Study the drawing (mm; zero at the part's minimum x, y, z) and answer. A direction names the side the tool comes from. Coordinates: 2 decimals unless noted, no trailing zeros. Write each loop counter-clockwise with the first axis right and the second up, starting at its lowest first coordinate (ties: lowest second). Pieces come first, ordered by that corner, then holes. Notation, with made-up numbers: (84.25, 75.25) -> (88.25, 75.25) arc R15 cw to (88.25, 81.25) -> close; hole circle Ø4 at (77, -17). An arc over 180 degrees is marked (long way). Write each question's results on one line, items separated by ' | '. Start each with the question number.
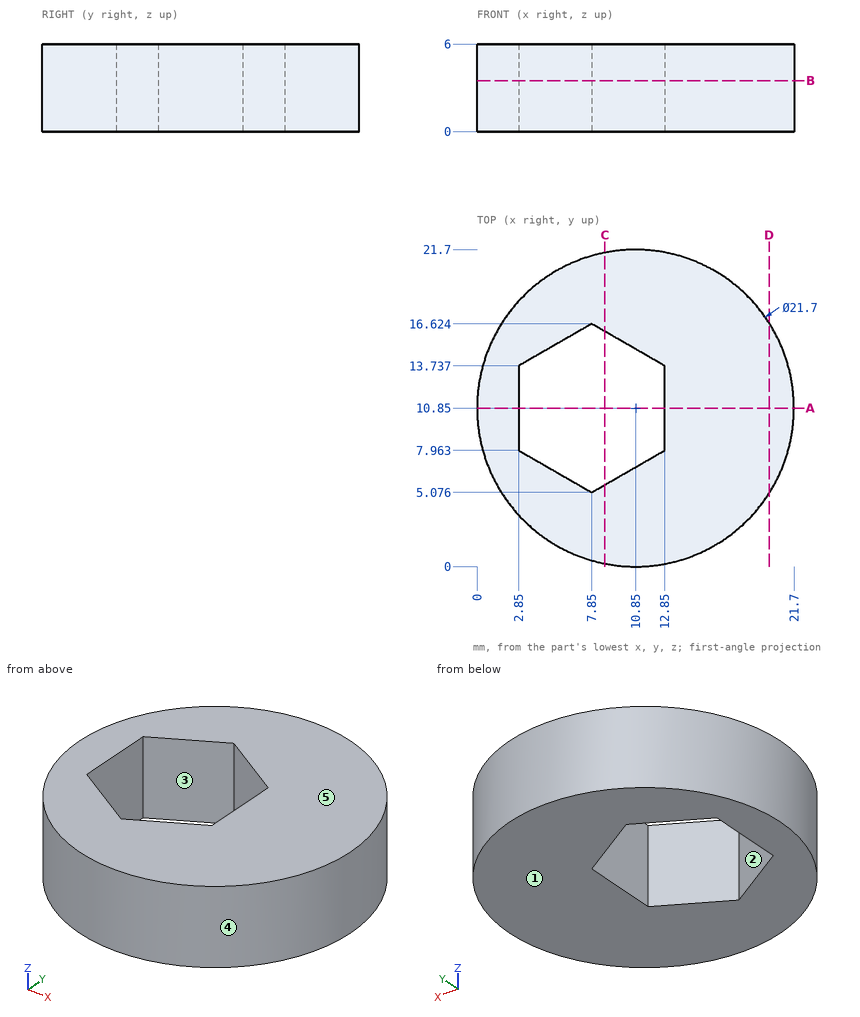
1. Determine the mould class of the marked faces 3, 4 and 5 for opening direction Y: pulls with the +Y half, pulls with the -Y half, needs draft (parallel to the pull), parting line crosses it, or undercut.
2. Find section C-C on x = 8.75. Give the vertices of the cut face in (y, z) (1 decimal).
3. Find section A-A on y = 10.85. Give the vertices of the cut face in (x, z), and give its area (3 significant figures).
4. Find the intervals of material crossed by L1, parallel to X at y = 15.75, z = 3.4 (1 decimal); L2, parallel to Y at x = 8.75, z = 0.45 (1 decimal); L3, parallel to X at y = 12, z = 4.5, in increasing order.
5. For the marked faces 1 and 2, determine the directions among +Z, -Z, +X, -X, +Y, -Y from which every point of the face is accessible in a straight line to the end or side of a thin tool.
6. Given pin 1 Ø3 at (y, z) = (16, 3.5) entering from +X; pin 2 Ø3 at (y, z) = (12.5, 4.5) entering from -X, each flat-ended and moving along its own axis, determine where each tip first touches the part or whether it passes through.
7. Find section B-B on z = 3.5. Give the vertices of the cut face in (x, y), and give its area (3 significant figures).
8. Find section D-D on x = 20. Give the vertices of the cut face in (y, z).
Ans:
1) face 3: undercut | face 4: parting line crosses it | face 5: needs draft
2) outline: (0.2, 0) -> (5.6, 0) -> (5.6, 6) -> (0.2, 6) -> close; (16.1, 0) -> (21.5, 0) -> (21.5, 6) -> (16.1, 6) -> close
3) outline: (0, 0) -> (2.85, 0) -> (2.85, 6) -> (0, 6) -> close; (12.85, 0) -> (21.7, 0) -> (21.7, 6) -> (12.85, 6) -> close | area: 70.2 mm²
4) L1: x = 1.2 to 6.3, 9.4 to 20.5 | L2: y = 0.2 to 5.6, 16.1 to 21.5 | L3: x = 0.06 to 2.85, 12.85 to 21.64
5) face 1: -Z, +X, -X, +Y, -Y | face 2: +Z, -Z
6) pin 1: stops at x = 21.07 | pin 2: stops at x = 0
7) outline: circle Ø21.7 at (10.85, 10.85); hole (2.85, 7.96) -> (7.85, 5.08) -> (12.85, 7.96) -> (12.85, 13.74) -> (7.85, 16.62) -> (2.85, 13.74) -> close | area: 283 mm²
8) outline: (5.02, 0) -> (16.68, 0) -> (16.68, 6) -> (5.02, 6) -> close
